Design review of the part built by this model. Coordinates are the model's own, in mm. Coordinates: 2 decimals unless noted, no trailing zeros. Loops run counter-clockwise (first coordinate to the right, second up) from the corner with the lowest first, then second, coordinate; pieces in that order, holes last. Notation, with made-up numbers: M -3.5,20 L 24.5,20 A27 ccw 24.5,48 Z; hole C 88,36 d5. An arc over 180 degrees is marked long. Write item = value, one per line. Start each with the question number.
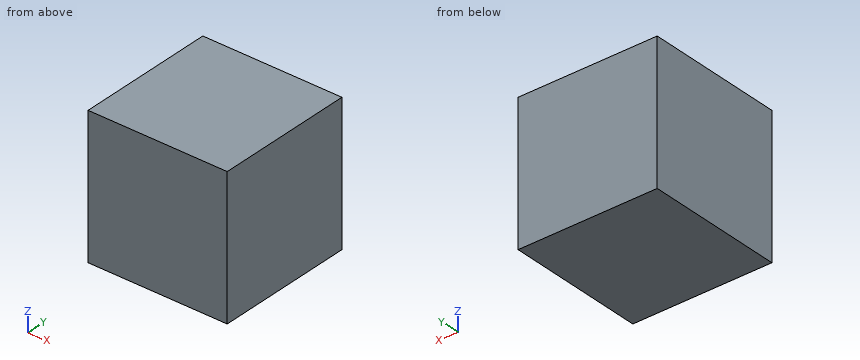
```python
from build123d import *

# Parameters (mm, degrees)
F3_W     = 76.2
F3_H     = 76.2
F3_W_2   = 71.12
F3_H_2   = 71.12
F4_DEPTH = 38.1
F2_W     = 76.2
F2_H     = 76.2
F2_W_2   = 71.12
F2_H_2   = 71.12
F5_DEPTH = 38.1


# Not quite as in the source:
# - a variable given as a bare number and used for a length is read in inches; the dataset says mm whatever the document's units were


with BuildPart() as f4:
    # F3 (on Right) → F4 (new body, symmetric)
    with BuildSketch(Plane.YZ):
        Rectangle(F3_W, F3_H)
        Rectangle(F3_W_2, F3_H_2, mode=Mode.SUBTRACT)
    extrude(amount=F4_DEPTH, both=True)

    # F2 (on Front) → F5 (join, symmetric)
    with BuildSketch(Plane.XZ):
        Rectangle(F2_W, F2_H)
        Rectangle(F2_W_2, F2_H_2, mode=Mode.SUBTRACT)
    extrude(amount=F5_DEPTH, both=True)


solid = f4.part
```
(1) Take a section at A-A (z = -21). State the section outline as (x, y) points, plus the area to 3 significant figures.
(2) To check wall thickness, follow L1, parallel to Z at x = 34, y = -1. State the ranges of the line that lie inside material, in increasing order.
Results list:
q1.outline = M -38.1,-38.1 L 38.1,-38.1 L 38.1,38.1 L -38.1,38.1 Z; hole M -35.56,-35.56 L 35.56,-35.56 L 35.56,35.56 L -35.56,35.56 Z
q1.area = 748 mm^2
q2.L1 = -38.1 to -35.56, 35.56 to 38.1
